```python
from build123d import *

# Parameters (mm, degrees)
SKETCH1_W               = 44.45
SKETCH1_H               = 44.45
SKETCH1_W_2             = 38.1
SKETCH1_H_2             = 38.1
BOSS_EXTRUDE1_DEPTH     = 1193.8
F_1_4_CLEARANCE_HOLE1_D = 6.7564


with BuildPart() as part:
    # Sketch1 → Boss-Extrude1 (new body)
    with BuildSketch(Plane(origin=(0, 0, 0), x_dir=(0, 0, -1), z_dir=(1, 0, 0))):
        Rectangle(SKETCH1_W, SKETCH1_H)
        Rectangle(SKETCH1_W_2, SKETCH1_H_2, mode=Mode.SUBTRACT)
    extrude(amount=BOSS_EXTRUDE1_DEPTH)

    # 1/4 Clearance Hole1 (through all)
    with Locations(Plane(origin=(0, 22.225, 0), x_dir=(1, 0, 0), z_dir=(0, 1, 0))):
        with Locations((311.15, 0), (146.05, 0), (19.05, 0), (1174.75, 0), (1047.75, 0), (882.65, 0)):
            Hole(F_1_4_CLEARANCE_HOLE1_D / 2)


solid = part.part
```
Work out the finished part from the listing and answer in its coordinate system (mm). A direction names the side the tool comes from. Give positions to 0.01 mm unless a question says otherwise; leave off trailing zeros. Write each loop counter-clockwise with the first axis right and the second up, starting at its lowest first coordinate (ties: lowest second). Pieces come first, ordered by that corner, then holes.
(1) The part is cut by section A-A on z = -11. Write down the section's boundary in (x, y) (3 decimals), plus the area to 3 significant figures.
Final values:
outline: (0, -22.225) - (1193.8, -22.225) - (1193.8, -19.05) - (0, -19.05) - close; (0, 19.05) - (1193.8, 19.05) - (1193.8, 22.225) - (0, 22.225) - close
area: 7,580 mm2
(2) Straight lines are drawn through the part: line 1 (Y direction, x = 728.5, z = 1.5) (3 decimals); line 2 (Z direction, x = 1174.75, y = -19.85) (3 decimals). For each, find the intervals that lie inside material, in ascending order.
Final values:
line 1: y = -22.225 to -19.05, 19.05 to 22.225
line 2: z = -22.225 to -3.378, 3.378 to 22.225
(3) Which of the six approach directions +Z, -Z, +X, -X, +Y, -Y give full straight-line access (tool end or side, diameter ignored) to faces 1 (the flat face through (589, -19.05, 0)), 2 (the flat face through (589, 22.225, 0))?
Final values:
face 1: +X, -X
face 2: +Z, -Z, +X, -X, +Y
(4) A flat-ended cylindrical pin translates along its axis: pin 1 Ø5.5 at (x, z) = (146.05, 0) entering from +Y. Find the tip coordinate at first contact, or state that the pin passes through.
Final values:
pin 1: passes through
(5) The mould has two halves that part along Z. Classify faces 3 (the flat face through (0, 0.3, -19.4)), 4 (the flat face through (589, 0, 19.05)), 5 (the flat face through (589, 0, 22.225)), 6 (the flat face through (589, 0, -19.05)): pulls with the +Z half, pulls with the -Z half, needs draft (parallel to the pull), parting line crosses it, or undercut.
Final values:
face 3: needs draft
face 4: undercut
face 5: pulls with the +Z half
face 6: undercut
(6) The part is cut by section B-B on x = 98.5. Write down the section's boundary in (y, z) (3 decimals).
Final values:
outline: (-22.225, -22.225) - (22.225, -22.225) - (22.225, 22.225) - (-22.225, 22.225) - close; hole (-19.05, -19.05) - (19.05, -19.05) - (19.05, 19.05) - (-19.05, 19.05) - close
